Source: CAD feature listing. Evaluate the final solid. Frame: model axes, mm. Face numbers are marked on the shaded views. Round coordinates to 2 decimals unless told otherwise and drop trailing zeros. Order: outer loops, then holes, each group sorted by start corner. A loop starts at its lowest first (then second) coordinate and runs counter-clockwise, first axis right, second up. Notation, with made-up numbers: (-18, 8.5) -> (-12, 8.5) arc R7 ccw to (-12, 13.5) -> close; hole circle Ø10 at (38.25, -18.5). An arc over 180 degrees is marked (long way). Answer as CSV lines item,"result". Start each with the question number.
(1) Section query B-B (z = -1.5). Output: boundary loops of the cut face in (x, y), plus the area to 3 significant figures.
(2) Pull-direction query (X, two-part tool) for the marked faces 1, 2, 3 and 4; classes: +X half, -X half, draft (parallel to the pull), parting line (faces both ways), or undercut.
(3) Contact query for flat-ended pins moving along their axis: P1, Ø1, axis at x = -228, z = 1, coming from the -Y side; P2, Ø5, axis at x = -206, z = 1, coming from the -Y side; P3, Ø6, axis at x = -231.5, z = 0.5, coming from the +Y side; P4, Ø3, axis at y = 345.5, z = -2.5, coming from the +X side. Output: stop coordinate, or through.
(4) Section query C-C (z = -3.75). Output: boundary loops of the cut face in (x, y).
(5) Section query A-A (z = 4.25). Output: boundary loops of the cut face in (x, y), plus the area to 3 significant figures.
(6) Line query: line 1 along Y through (x, z) = (-212.5, 2.25); line 2 along Y through (x, z) = (-219.5, 0.5); line 3 along X through (y, z) = (361, -4). Output: solid intervals per line, ascending. Write a range as from..to.
```python
from build123d import *

# Parameters (mm, degrees)
CABEZA_PROFILE_R  = 5
VASTAGO_PROFILE_R = 3
TUERCA_PROFILE_R  = 5


with BuildPart() as part:
    # Cabeza: sweep along a curve in space
    with BuildLine() as cabeza_path:
        Line((-234.974862986, 359.135649617, 0), (-238.177480086, 361.53215618, 0))
    # Cabeza profile (on start of the path) → Cabeza (sweep)
    with BuildSketch(Plane(origin=(-234.974862986, 359.135649617, 0), x_dir=(-0.5991266409502999, -0.8006542750173826, 0), z_dir=(-0.8006542750173826, 0.5991266409502999, 0))):
        Circle(CABEZA_PROFILE_R)
    sweep(path=cabeza_path.line)

    # Vastago: sweep along a curve in space
    with BuildLine() as vastago_path:
        Line((-202.948691985, 335.170583979, 0), (-234.974862986, 359.135649617, 0))
    # Vastago profile (on start of the path) → Vastago (sweep)
    with BuildSketch(Plane(origin=(-202.948691985, 335.170583979, 0), x_dir=(-0.5991266409502972, -0.8006542750173845, 0), z_dir=(-0.8006542750173845, 0.5991266409502972, 0))):
        Circle(VASTAGO_PROFILE_R)
    sweep(path=vastago_path.line)

    # Tuerca: sweep along a curve in space
    with BuildLine() as tuerca_path:
        Line((-205.35065481, 336.967963901, 0), (-210.15458046, 340.562723747, 0))
    # Tuerca profile (on start of the path) → Tuerca (sweep)
    with BuildSketch(Plane(origin=(-205.35065481, 336.967963901, 0), x_dir=(-0.5991266409502919, -0.8006542750173886, 0), z_dir=(-0.8006542750173886, 0.5991266409502919, 0))):
        Circle(TUERCA_PROFILE_R)
    sweep(path=tuerca_path.line)


solid = part.part
```
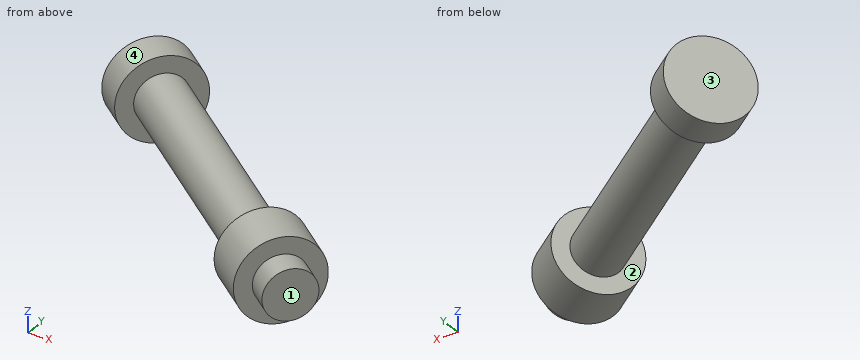
Answer block:
1,outline,"(-241.04, 357.71) -> (-237.83, 355.32) -> (-236.53, 357.06) -> (-211.71, 338.48) -> (-213.01, 336.74) -> (-208.21, 333.15) -> (-206.91, 334.89) -> (-204.51, 333.09) -> (-201.39, 337.25) -> (-203.79, 339.05) -> (-202.49, 340.79) -> (-207.3, 344.38) -> (-208.6, 342.64) -> (-233.42, 361.22) -> (-232.12, 362.95) -> (-235.32, 365.35) -> close"
1,area,"272 mm2"
2,face 1,"+X half"
2,face 2,"undercut"
2,face 3,"-X half"
2,face 4,"parting line"
3,P1,"y = 349.96"
3,P2,"y = 332.77"
3,P3,"y = 365.01"
3,P4,"x = -207.19"
4,outline,"(-240.16, 358.88) -> (-236.96, 356.49) -> (-232.99, 361.78) -> (-236.2, 364.18) -> close; (-212.14, 337.91) -> (-207.33, 334.32) -> (-203.37, 339.62) -> (-208.17, 343.21) -> close"
5,outline,"(-239.76, 359.42) -> (-236.55, 357.03) -> (-233.4, 361.24) -> (-236.6, 363.64) -> close; (-211.73, 338.45) -> (-206.93, 334.86) -> (-203.77, 339.08) -> (-208.58, 342.67) -> close"
5,area,"52.7 mm2"
6,line 1,"336.74..337.43, 339.84..344.8"
6,line 2,"343.86..351.25"
6,line 3,"-238.58..-233.58"
